Part model, mm, in its own coordinate system. Give positions to 0.01 mm unless a question says otherwise; leave off trailing zeros. Write each loop counter-clockwise with the first axis right and the second up, starting at its lowest first coordinate (ties: lowest second). Pieces come first, ordered by that corner, then holes.
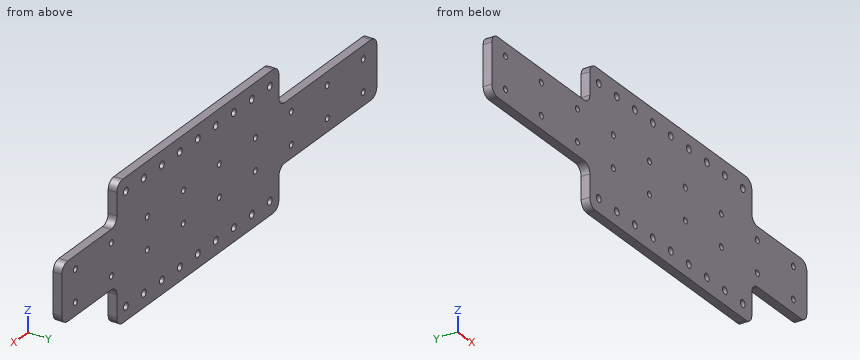
```python
from build123d import *

# Parameters (mm, degrees)
SKETCH7_W           = 350
SKETCH7_H           = 42
BOSS_EXTRUDE3_DEPTH = 6.35
SKETCH2_R           = 2.15
CUT_EXTRUDE1_DEPTH  = 177.369845779
SKETCH1_W           = 180
SKETCH1_H           = 29.00074531
SKETCH1_H_2         = 28.99925469
BOSS_EXTRUDE4_DEPTH = 6.35
SKETCH3_R           = 2.65
CUT_EXTRUDE2_DEPTH  = 183.113692598
FILLET2_R           = 6.35


with BuildPart() as part:
    # Sketch7 → Boss-Extrude3 (new body)
    with BuildSketch(Plane(origin=(0, 0, 0), x_dir=(1, 0, 0), z_dir=(0, 1, 0))):
        Rectangle(SKETCH7_W, SKETCH7_H)
    extrude(amount=-BOSS_EXTRUDE3_DEPTH)

    # Sketch2 → Cut-Extrude1 (cut, through all)
    with BuildSketch(Plane(origin=(0, 0, 0), x_dir=(1, 0, 0), z_dir=(0, 1, 0))):
        with Locations(Location((120, 11.5, 0), (0, 0, 270))):
            Circle(SKETCH2_R)
        with Locations(Location((120, -11.5, 0), (0, 0, 90))):
            Circle(SKETCH2_R)
        with Locations(Location((80, 11.5, 0), (0, 0, 270))):
            Circle(SKETCH2_R)
        with Locations(Location((160, 11.5, 0), (0, 0, 270))):
            Circle(SKETCH2_R)
        with Locations(Location((80, -11.5, 0), (0, 0, 90))):
            Circle(SKETCH2_R)
        with Locations(Location((160, -11.5, 0), (0, 0, 90))):
            Circle(SKETCH2_R)
        with Locations(Location((40, 11.5, 0), (0, 0, 270))):
            Circle(SKETCH2_R)
        with Locations(Location((40, -11.5, 0), (0, 0, 90))):
            Circle(SKETCH2_R)
        with Locations(Location((0, 11.5, 0), (0, 0, 270))):
            Circle(SKETCH2_R)
        with Locations(Location((0, -11.5, 0), (0, 0, 90))):
            Circle(SKETCH2_R)
        with Locations(Location((-40, 11.5, 0), (0, 0, 270))):
            Circle(SKETCH2_R)
        with Locations(Location((-40, -11.5, 0), (0, 0, 90))):
            Circle(SKETCH2_R)
        with Locations(Location((-80, 11.5, 0), (0, 0, 270))):
            Circle(SKETCH2_R)
        with Locations(Location((-80, -11.5, 0), (0, 0, 90))):
            Circle(SKETCH2_R)
        with Locations(Location((-120, 11.5, 0), (0, 0, 270))):
            Circle(SKETCH2_R)
        with Locations(Location((-120, -11.5, 0), (0, 0, 90))):
            Circle(SKETCH2_R)
        with Locations(Location((-160, 11.5, 0), (0, 0, 270))):
            Circle(SKETCH2_R)
        with Locations(Location((-160, -11.5, 0), (0, 0, 90))):
            Circle(SKETCH2_R)
    extrude(amount=-CUT_EXTRUDE1_DEPTH, mode=Mode.SUBTRACT)

    # Sketch1 → Boss-Extrude4 (add, through all)
    with BuildSketch(Plane(origin=(0, 0, 0), x_dir=(1, 0, 0), z_dir=(0, 1, 0))):
        with Locations((23.874417882, -35.500372655)):
            Rectangle(SKETCH1_W, SKETCH1_H)
        with Locations((23.874417882, 35.499627345)):
            Rectangle(SKETCH1_W, SKETCH1_H_2)
    extrude(amount=-BOSS_EXTRUDE4_DEPTH)

    # Sketch3 → Cut-Extrude2 (cut, through all)
    with BuildSketch(Plane(origin=(0, 0, 0), x_dir=(1, 0, 0), z_dir=(0, 1, 0))):
        with Locations(Location((23.874417882, 39.99925469, 0), (0, 0, 270))):
            Circle(SKETCH3_R)
        with Locations(Location((43.874417882, 39.99925469, 0), (0, 0, 270))):
            Circle(SKETCH3_R)
        with Locations(Location((63.874417882, 39.99925469, 0), (0, 0, 270))):
            Circle(SKETCH3_R)
        with Locations(Location((103.874417882, 39.99925469, 0), (0, 0, 270))):
            Circle(SKETCH3_R)
        with Locations(Location((-36.125582118, 39.99925469, 0), (0, 0, 270))):
            Circle(SKETCH3_R)
        with Locations(Location((83.874417882, 39.99925469, 0), (0, 0, 270))):
            Circle(SKETCH3_R)
        with Locations(Location((-56.125582118, 39.99925469, 0), (0, 0, 270))):
            Circle(SKETCH3_R)
        with Locations(Location((-16.125582118, 39.99925469, 0), (0, 0, 270))):
            Circle(SKETCH3_R)
        with Locations(Location((3.874417882, 39.99925469, 0), (0, 0, 270))):
            Circle(SKETCH3_R)
        with Locations(Location((3.874417882, -40.00074531, 0), (0, 0, 270))):
            Circle(SKETCH3_R)
        with Locations(Location((-16.125582118, -40.00074531, 0), (0, 0, 270))):
            Circle(SKETCH3_R)
        with Locations(Location((-56.125582118, -40.00074531, 0), (0, 0, 270))):
            Circle(SKETCH3_R)
        with Locations(Location((83.874417882, -40.00074531, 0), (0, 0, 270))):
            Circle(SKETCH3_R)
        with Locations(Location((-36.125582118, -40.00074531, 0), (0, 0, 270))):
            Circle(SKETCH3_R)
        with Locations(Location((103.874417882, -40.00074531, 0), (0, 0, 270))):
            Circle(SKETCH3_R)
        with Locations(Location((63.874417882, -40.00074531, 0), (0, 0, 270))):
            Circle(SKETCH3_R)
        with Locations(Location((43.874417882, -40.00074531, 0), (0, 0, 270))):
            Circle(SKETCH3_R)
        with Locations(Location((23.874417882, -40.00074531, 0), (0, 0, 270))):
            Circle(SKETCH3_R)
    extrude(amount=-CUT_EXTRUDE2_DEPTH, mode=Mode.SUBTRACT)

    # Fillet2
    fillet2_edges = [part.edges().sort_by_distance(p)[0] for p in [
        (113.874417882, -3.175, 50.00074531),
        (113.874417882, -3.175, 21),
        (113.874417882, -3.175, -21),
        (113.874417882, -3.175, -49.99925469),
        (-66.125582118, -3.175, -49.99925469),
        (-66.125582118, -3.175, -21),
        (-175, -3.175, -21),
        (-175, -3.175, 21),
        (-66.125582118, -3.175, 50.00074531),
        (-66.125582118, -3.175, 21),
        (175, -3.175, 21),
        (175, -3.175, -21),
    ]]
    fillet(fillet2_edges, radius=FILLET2_R)


solid = part.part
```
1) Saw through at A-A, the plane x = 146. Write the cut outline in (y, z).
Answers follow:
outline: (-6.35, -21) - (0, -21) - (0, 21) - (-6.35, 21) - close
2) Saw through at B-B, the plane y = -1.5. Count the separate pieces of the cut face and the enclosed holes in it, then the cut area to 3 significant figures.
Answers follow:
separate pieces: 1
enclosed holes: 36
area: 24,400 mm2
3) Wall check: L1, parallel to Z at x = 26, y = -1.5; L2, parallel to X at y = -4.5, z = 35.5; L3, parallel to Z at x = -152, y = -3.25. Give the ranges that are in metal, low to high.
Answers follow:
L1: z = -50 to -41.58, -38.42 to 38.42, 41.58 to 50
L2: x = -66.13 to 113.87
L3: z = -21 to 21
4) Pin check, flat tips, straight feed: pin 1 Ø3 at (y, z) = (-1.5, 16.5) entering from +X; pin 2 Ø3 at (y, z) = (-2, -32) entering from +X; pin 3 Ø1.9 at (x, y) = (139, -2.5) entering from -Z. Stop position of each tip, or through.
Answers follow:
pin 1: stops at x = 174.99
pin 2: stops at x = 113.87
pin 3: stops at z = -21
